Autodesk Inventor part; units mm, degrees
ref_plane "作業平面1" through (2.15, -10, 1000) normal (0, 0, 1) x (1, 0, 0)
ref_plane "YZ Plane" through (0, 0, 0) normal (1, 0, 0) x (0, 1, 0)
ref_plane "XZ Plane" through (0, 0, 0) normal (0, 1, 0) x (-1, 0, 0)
ref_plane "作業平面1" through (2.15, -10, 1000) normal (0, 0, 1) x (1, 0, 0)
sketch "スケッチ1" plane through (2.15, -10, 1000) normal (0, 0, 1) x (1, 0, 0)
  line L0 (6.35, 12.15) -> (7.85, 12.15)
  line L1 (7.85, 12.15) -> (7.85, 19.4936)
  arc A0 (7.85, 19.4936) -> (7.3372, 19.9934) centre (7.35, 19.4936) ccw
  arc A1 (7.3372, 19.9934) -> (-12.1434, 0.5128) centre (7.85, 0) ccw
  arc A2 (-12.1434, 0.5128) -> (-11.6436, 0) centre (-11.6436, 0.5) ccw
  line L2 (-11.6436, 0) -> (-4.3, 0)
  line L3 (-4.3, 0) -> (-4.3, 1.5)
  line L4 (-4.3, 1.5) -> (-6.3, 1.5)
  line L5 (-6.3, 1.5) -> (-6.3, 5.2)
  line L6 (-6.3, 5.2) -> (-4.3, 5.2)
  line L7 (-4.3, 5.2) -> (-4.3, 7)
  line L8 (-4.3, 7) -> (0, 7)
  line L9 (0, 7) -> (0, 5.2)
  line L10 (0, 5.2) -> (2, 5.2)
  line L11 (2, 5.2) -> (2, 1.5)
  line L12 (2, 1.5) -> (0, 1.5)
  line L13 (0, 1.5) -> (0, 0)
  line L14 (0, 0) -> (7.35, 0)
  arc A3 (7.35, 0) -> (7.85, 0.5) centre (7.35, 0.5) ccw
  line L15 (7.85, 0.5) -> (7.85, 7.85)
  line L16 (7.85, 7.85) -> (6.35, 7.85)
  line L17 (6.35, 7.85) -> (6.35, 5.85)
  line L18 (6.35, 5.85) -> (2.65, 5.85)
  line L19 (2.65, 5.85) -> (2.65, 7.85)
  line L20 (2.65, 7.85) -> (0.85, 7.85)
  line L21 (0.85, 7.85) -> (0.85, 12.15)
  line L22 (0.85, 12.15) -> (2.65, 12.15)
  line L23 (2.65, 12.15) -> (2.65, 14.15)
  line L24 (2.65, 14.15) -> (6.35, 14.15)
  line L25 (6.35, 14.15) -> (6.35, 12.15)
  circle A4 centre (4.85, 3) radius 2
  circle A5 centre (-9.15, 3) radius 2
  circle A6 centre (4.85, 17) radius 2
  circle A7 centre (-2.15, 10) radius 1.65
extrude "押し出し1" add sketch "スケッチ1" along normal blind 330
properties part number "AFSR-2020-4-1000"
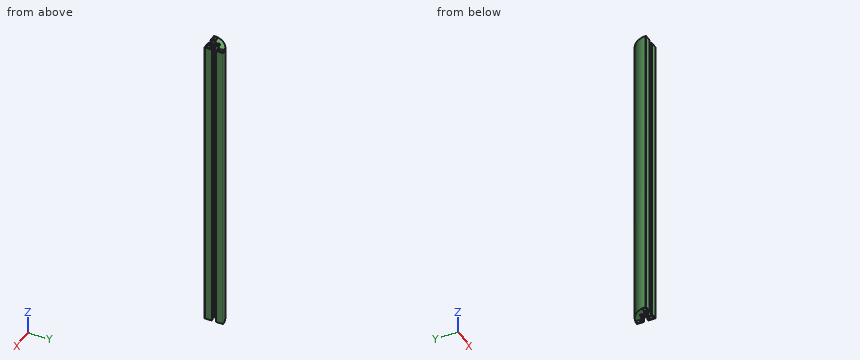
The model under review builds one solid part; all positions refer to its coordinate system, in mm. Round coordinates to 2 decimals unless told otherwise and drop trailing zeros.
Item 1: Clearance check with flat-ended pins moving along their axes: pin 1 Ø1.4 at (y, z) = (-3.5, 1188) entering from -X; pin 2 Ø4 at (y, z) = (-6, 1231.5) entering from -X; pin 3 Ø10 at (y, z) = (1.5, 1057.5) entering from -X; pin 4 Ø5 at (x, y) = (7, -7) entering from -Z. State where each tip first meets the part, or that it passes through.
Determined:
pin 1: stops at x = -9.14
pin 2: stops at x = -9.9
pin 3: stops at x = -8.91
pin 4: stops at z = 1000
Item 2: For line 1 (Y direction, x = 7.25, z = 1258.5); line 2 (X direction, y = -2.5, z = 1050); line 3 (X direction, y = 3.25, z = 1194.5), list the stretches that pass through material, from the lowest coordinate up.
Determined:
line 1: y = -10 to -8.98, -5.02 to -4.15, 4.15 to 5.02, 8.98 to 9.81
line 2: x = -8.54 to 4.8, 8.5 to 10
line 3: x = -4.98 to 4.8, 8.5 to 10
Item 3: Take a section at A-A (z = 1200). Give the number of separate pieces and of enclosed holes in the cut face, then the cut area to 3 significant figures.
Determined:
separate pieces: 1
enclosed holes: 4
area: 178 mm2
